from build123d import *

# Parameters (mm, degrees)
F2_DEPTH  = 4
F3_W      = 4
F3_H      = 30
F4_DEPTH  = 6
F5_SIZE   = 16
F6_SIZE   = 2
F7_SIZE   = 4
F8_W      = 4
F8_H      = 92
F9_DEPTH  = 11
F10_R     = 4.5
F11_DEPTH = 2.4
F12_R     = 2.3
F13_DEPTH = 4
F14_SIZE  = 4
F15_SIZE  = 1.99999


# Not quite as in the source:
# - a fillet or chamfer is up to 0.001 mm smaller than in the source, because OpenCascade refuses the exact size


with BuildPart() as f2:
    # F1 (on Top) → F2 (new body)
    with BuildSketch(Plane.XY):
        Polygon((10, 46), (-4, 46), (-4, -46), (10, -46), (10, -10), (76.5, -10), (76.5, 20), (10, 20), align=None)
    extrude(amount=F2_DEPTH)

    # F3 (on face) → F4 (join)
    with BuildSketch(Plane.XY.offset(4)):
        with Locations((74.5, 5)):
            Rectangle(F3_W, F3_H)
    extrude(amount=F4_DEPTH)

    # F5
    f5_edges = [f2.edges().sort_by_distance(p)[0] for p in [
        (10, 20, 2),
        (10, -10, 2),
    ]]
    chamfer(f5_edges, length=F5_SIZE)

    # F6
    f6_edges = [f2.edges().sort_by_distance(p)[0] for p in [
        (72.5, 5, 10),
    ]]
    chamfer(f6_edges, length=F6_SIZE)

    # F7
    f7_edges = [f2.edges().sort_by_distance(p)[0] for p in [
        (10, -46, 2),
        (10, 46, 2),
    ]]
    chamfer(f7_edges, length=F7_SIZE)

    # F8 (on face) → F9 (join)
    with BuildSketch(Plane.XY.offset(4)):
        with Locations((-2, 0)):
            Rectangle(F8_W, F8_H)
    extrude(amount=F9_DEPTH)

    # F10 (on face) → F11 (cut)
    with BuildSketch(Plane.YZ):
        with Locations((-38, 8.5)):
            Circle(F10_R)
        with Locations((38, 8.5)):
            Circle(F10_R)
    extrude(amount=-F11_DEPTH, mode=Mode.SUBTRACT)

    # F12 (on face) → F13 (cut, through all)
    with BuildSketch(Plane(origin=(-4, 0, 0), x_dir=(0, -1, 0), z_dir=(-1, 0, 0))):
        with Locations((-38, 8.5)):
            Circle(F12_R)
        with Locations((38, 8.5)):
            Circle(F12_R)
    extrude(amount=-F13_DEPTH, mode=Mode.SUBTRACT)

    # F14
    f14_edges = [f2.edges().sort_by_distance(p)[0] for p in [
        (-2, -46, 15),
        (-2, 46, 15),
    ]]
    chamfer(f14_edges, length=F14_SIZE)

    # F15 (size 2 in the source; OpenCascade refuses exactly that, so slightly less here)
    f15_edges = [f2.edges().sort_by_distance(p)[0] for p in [
        (0, 0, 15),
    ]]
    chamfer(f15_edges, length=F15_SIZE)


solid = f2.part
Could you check a few things on this model? Use its own coordinates, in mm. A direction names the side the tool comes from. Coordinates: 2 decimals unless noted, no trailing zeros. Order: outer loops, then holes, each group sorted by start corner. A loop starts at its lowest first (then second) coordinate and runs counter-clockwise, first axis right, second up.
Q1. Please list where these lines run through material, in increasing order: L1, parallel to Y at x = -0.75, z = 8.5; L2, parallel to Z at x = -3, y = -38; L3, parallel to Z at x = 31.5, y = 17.5.
Q2. Suppose I cut it at B-B on z = 1.25. Please give me the cut outline in (x, y).
Q3. Suppose I cut it at C-C on x = 47. Please give me the cut outline in (y, z).
Q4. Suppose I cut it at A-A on y = 28. Please give me the cut outline in (x, z), and give its area (3 significant figures).
Q5. Thinking about a two-plate mould opening in X: for faces 6 (the flat face through (8, 44, 2)), 7 (the flat face through (51, -10, 3)), 8 (the flat face through (0, -1, 8)), 9 (the flat face through (72.5, 5, 6)), which applies, released by +X, released by -X, zero draft, split by the parting line, or undercut?
Q6. Suppose I cut it at D-D on y = -14. Please give me the cut outline in (x, z).
Q7. Which directions (+Z, -Z, +X, -X, +Y, -Y) give clear straight access to the entire face, cutting with the end or side of a thin tool? Please do faces 1 (the flat face through (10, -34, 2)), 2 (the flat face through (75, 5, 10)), 3 (the flat face through (-3, 1, 15)), 4 (the flat face through (-2, -44, 13)), 5 (the cylindrical face through (-1.183, 42.292, 9.852)).
Q8. Will these pins go through, and if not, where does the flat tip stop? pin 1 (5 mm diameter, centred on x = 59.5, z = 7, fed in from +Y); pin 2 (7.5 mm diameter, centred on y = 38, z = 8.5, fed in from +X); pin 3 (7 mm diameter, centred on y = 40, z = 8, fed in from +X); pin 4 (8 mm diameter, centred on x = 13.5, y = 26.5, fed in from +Z).
Answer:
1. L1: y = -46 to -42.5, -33.5 to 33.5, 42.5 to 46
1. L2: z = 0 to 6.2, 10.8 to 15
1. L3: z = 0 to 4
2. outline: (-4, -46) - (6, -46) - (10, -42) - (10, -26) - (26, -10) - (76.5, -10) - (76.5, 20) - (26, 20) - (10, 36) - (10, 42) - (6, 46) - (-4, 46) - close
3. outline: (-10, 0) - (20, 0) - (20, 4) - (-10, 4) - close
4. outline: (-4, 0) - (18, 0) - (18, 4) - (0, 4) - (0, 13) - (-2, 15) - (-4, 15) - close
4. area: 130 mm2
5. face 6: released by +X
5. face 7: zero draft
5. face 8: undercut
5. face 9: undercut
6. outline: (-4, 0) - (22, 0) - (22, 4) - (0, 4) - (0, 13) - (-2, 15) - (-4, 15) - close
7. face 1: +Z, -Z, +X, -Y
7. face 2: +Z, +X, +Y, -Y
7. face 3: +Z, +X, -X, +Y, -Y
7. face 4: +Z, +X, -X, -Y
7. face 5: +X
8. pin 1: passes through
8. pin 2: stops at x = -2.4
8. pin 3: stops at x = 0
8. pin 4: stops at z = 4
